Work out the finished part from the listing and answer in its coordinate system (mm). A direction names the side the tool comes from. Coordinates: 2 decimals unless noted, no trailing zeros. Order: outer loops, then holes, each group sorted by start corner. A loop starts at its lowest first (then second) coordinate and runs counter-clockwise, first axis right, second up. Notation, with made-up numbers: (8.5, -16) -> (66.5, -16) arc R29 ccw to (66.5, 5) -> close; hole circle Ø5 at (23.5, 49). An arc over 180 degrees is marked (long way). Write item = value, one per line. Start each with the question number.
Q1. Which of the six approach directions +Z, -Z, +X, -X, +Y, -Y give full straight-line access (tool end or side, diameter ignored) to faces 5 (the flat face through (-3.008, 6.854, 3.091)), 6 (the conical face through (-8.19, 2.214, 1.474))?
Q2. Flat-ended cylindrical pins translate along their axes: pin 1 (3 mm diameter, centred on x = -1.5, z = 2.5, fed in from -Y); pin 2 (5 mm diameter, centred on x = 0, y = 0, fed in from +Z); pin 3 (3 mm diameter, centred on x = -8, z = 1.5, fed in from -Y); pin 4 (3 mm diameter, centred on x = -3.5, z = 4.5, fed in from -Y). Find the tip coordinate at first contact, or state that the pin passes through.
Q3. For a pull along Y with two mould halves and no side action, classify faces 1 (the flat face through (1.3, 1.2, 2)), 2 (the cylindrical face through (-4.77, 2.74, 2.54)), 3 (the cylindrical face through (-9.664, -2.571, 3.981)), 4 (the flat face through (-0.81, 7.38, 3.09)) as +Y half, -Y half, draft (parallel to the pull), parting line (faces both ways), or undercut.
Q4. The part is cut by section B-B, the plane y = 7.25. Count the separate pieces of the cut face and the enclosed holes in it, plus the area to 3 significant figures.
Q5. The part is cut by section A-A, the plane x = 0. Determine the outline of the cut face in (y, z), plus the area to 3 significant figures.
Q6. Straight lines are drawn through the part: L1, parallel to X at y = 0, z = 1.55; L2, parallel to X at y = 5.75, z = 2.7. For each, find the intervals that lie inside material, in ascending order. Write a range as from..to.
```python
from build123d import *

# Parameters (mm, degrees)
SKETCH_R           = 10
SKETCH_R_2         = 1.55
PAD_DEPTH          = 5
POCKET_DEPTH       = 3
CHAMFER_SIZE       = 2.99
POCKET001_DEPTH    = 7
POLARPATTERN_COUNT = 12


with BuildPart() as part:
    # Sketch → Pad (new body)
    with BuildSketch(Plane.XY):
        Circle(SKETCH_R)
        Circle(SKETCH_R_2, mode=Mode.SUBTRACT)
    extrude(amount=PAD_DEPTH)

    # Sketch001 (on Face4 of Pad) → Pocket (cut)
    with BuildSketch(Plane.XY.offset(5)):
        Polygon((-1.55, -2.684679), (1.55, -2.684679), (3.1, 0), (1.55, 2.684679), (-1.55, 2.684679), (-3.1, 0), align=None)
    extrude(amount=-POCKET_DEPTH, mode=Mode.SUBTRACT)

    # Chamfer
    chamfer_edges = [part.edges().sort_by_distance(p)[0] for p in [
        (-10, 0, 0),
    ]]
    chamfer(chamfer_edges, length=CHAMFER_SIZE)

    # Sketch002 (on Face3 of Pocket) → Pocket001 (cut)
    with BuildSketch(Plane.XY.offset(5)):
        with BuildLine():
            ThreePointArc((-0.467595, 5.822927), (0, 5.5), (0.467595, 5.822927))
            Line((2, 12.822927), (0.467595, 5.822927))
            Line((-2, 12.822927), (2, 12.822927))
            Line((-0.467595, 5.822927), (-2, 12.822927))
        make_face()
    pocket001 = extrude(amount=-POCKET001_DEPTH, mode=Mode.SUBTRACT)

    # PolarPattern: Pocket001 ×12 about axis
    polarpattern_axis = Axis((0, 0, 5), (0, 0, 1))
    for i in range(1, POLARPATTERN_COUNT):
        add(pocket001.rotate(polarpattern_axis, i * 360 / POLARPATTERN_COUNT), mode=Mode.SUBTRACT)


solid = part.part
```
Model answer:
q1.face_5 = +Z, -Z
q1.face_6 = -Z, -X, +Y
q2.pin_1 = -9.91
q2.pin_2 = 2
q2.pin_3 = -6.62
q2.pin_4 = -9.8
q3.face_1 = undercut
q3.face_2 = undercut
q3.face_3 = -Y half
q3.face_4 = +Y half
q4.separate_pieces = 4
q4.enclosed_holes = 0
q4.area = 27.7 mm2
q5.outline = (-5.5, 0) -> (-1.55, 0) -> (-1.55, 2) -> (-2.68, 2) -> (-2.68, 5) -> (-5.5, 5) -> close; (1.55, 0) -> (5.5, 0) -> (5.5, 5) -> (2.68, 5) -> (2.68, 2) -> (1.55, 2) -> close
q5.area = 32.7 mm2
q6.L1 = -5.5..-1.55, 1.55..5.5
q6.L2 = -7.48..-4.17, -2.66..-0.43, 0.43..2.66, 4.17..7.48
